For this review, take the finished solid that the model builds, in its own axes (mm). Face numbers are marked on the shaded views. A direction names the side the tool comes from. Round coordinates to 2 decimals unless told otherwise and drop trailing zeros. Order: outer loops, then holes, each group sorted by start corner. A loop starts at its lowest first (then second) coordinate and runs counter-clockwise, first axis right, second up. Notation, with made-up numbers: M 84.25,-30.5 L 132.25,-30.5 A19 cw 132.25,-24.5 Z; hole C 30.5,48.25 d10. An arc over 180 degrees is marked long. Put each result on its own line as item: value.
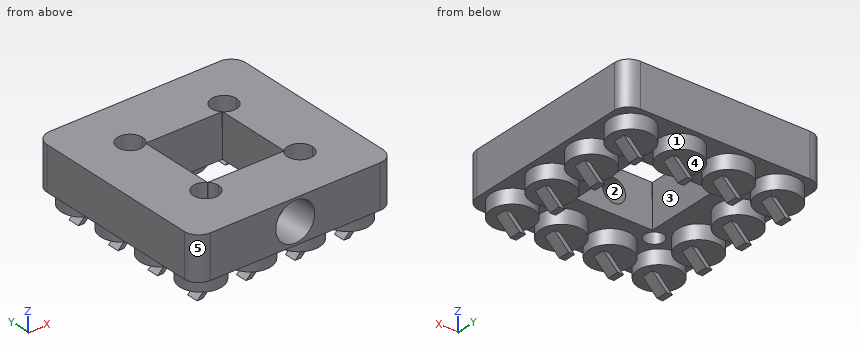
Autodesk Inventor part; units mm, degrees
ref_plane "YZ Plane" through (0, 0, 0) normal (1, 0, 0) x (0, 1, 0)
ref_plane "XZ Plane" through (0, 0, 0) normal (0, 1, 0) x (-1, 0, 0)
ref_plane "XY Plane" through (0, 0, 0) normal (0, 0, 1) x (1, 0, 0)
sketch "Sketch1" plane through (0, 0, 0) normal (0, 0, 1) x (1, 0, 0)
  circle A0 centre (16.335, -16.335) radius 2.25
  circle A1 centre (-16.335, 16.335) radius 2.25
  circle A2 centre (16.335, 16.335) radius 2.25
  circle A3 centre (-16.335, -16.335) radius 2.25
  line L0 (-13.335, 13.335) -> (13.335, 13.335)
  line L1 (13.335, 13.335) -> (13.335, -13.335)
  line L2 (13.335, -13.335) -> (-13.335, -13.335)
  line L3 (-13.335, -13.335) -> (-13.335, 13.335)
  circle A4 centre (25.5, -25.5) radius 8.0375
  circle A5 centre (8.5, -25.5) radius 8.0375
  circle A6 centre (-25.5, -25.5) radius 8.0375
  circle A7 centre (-8.5, -25.5) radius 8.0375
  circle A8 centre (25.5, -8.5) radius 8.0375
  circle A9 centre (25.5, 8.5) radius 8.0375
  circle A10 centre (-25.5, -8.5) radius 8.0375
  circle A11 centre (-25.5, 8.5) radius 8.0375
  circle A12 centre (25.5, 25.5) radius 8.0375
  circle A13 centre (8.5, 25.5) radius 8.0375
  circle A14 centre (-25.5, 25.5) radius 8.0375
  circle A15 centre (-8.5, 25.5) radius 8.0375
  arc A16 (29.5, -34.5) -> (34.5, -29.5) centre (29.5, -29.5) ccw
  line L4 (34.5, -29.5) -> (34.5, 29.5)
  arc A17 (34.5, 29.5) -> (29.5, 34.5) centre (29.5, 29.5) ccw
  line L5 (29.5, 34.5) -> (-29.5, 34.5)
  arc A18 (-29.5, 34.5) -> (-34.5, 29.5) centre (-29.5, 29.5) ccw
  line L6 (-34.5, 29.5) -> (-34.5, -29.5)
  arc A19 (-34.5, -29.5) -> (-29.5, -34.5) centre (-29.5, -29.5) ccw
  line L7 (-29.5, -34.5) -> (29.5, -34.5)
  circle A20 centre (-25.5, -25.5) radius 7.2875
  circle A21 centre (-8.5, -25.5) radius 7.2875
  circle A22 centre (8.5, -25.5) radius 7.2875
  circle A23 centre (25.5, -25.5) radius 7.2875
  circle A24 centre (-25.5, -8.5) radius 7.2875
  circle A25 centre (25.5, -8.5) radius 7.2875
  circle A26 centre (-25.5, 8.5) radius 7.2875
  circle A27 centre (25.5, 8.5) radius 7.2875
  circle A28 centre (-25.5, 25.5) radius 7.2875
  circle A29 centre (-8.5, 25.5) radius 7.2875
  circle A30 centre (8.5, 25.5) radius 7.2875
  circle A31 centre (25.5, 25.5) radius 7.2875
  point P0 (0, 0)
  dimension "d40" = 0.75
  dimension "d41" = 0.75
  dimension "d42" = 0.75
  dimension "d43" = 0.75
  dimension "d44" = 0.75
  dimension "d45" = 0.75
  dimension "d46" = 0.75
  dimension "d47" = 0.75
  dimension "d48" = 0.75
  dimension "d49" = 0.75
  dimension "d50" = 0.75
  dimension "d51" = 0.75
extrude "Extrusion1" add sketch "Sketch1" against normal blind 5 contours A20 | A21 | A22 | A23 | A24 | A25 | A26 | A27 | A28 | A29 | A30 | A31
ref_plane "Work Plane1" through (0, 0, 0) normal (0, 0, 1) x (1, 0, 0)
sketch "Sketch2" plane through (0, 0, 0) normal (0, 0, 1) x (1, 0, 0)
  circle A0 centre (16.335, -16.335) radius 2.25
  circle A1 centre (-16.335, 16.335) radius 2.25
  circle A2 centre (16.335, 16.335) radius 2.25
  circle A3 centre (-16.335, -16.335) radius 2.25
  line L0 (-13.335, 13.335) -> (13.335, 13.335)
  line L1 (13.335, 13.335) -> (13.335, -13.335)
  line L2 (13.335, -13.335) -> (-13.335, -13.335)
  line L3 (-13.335, -13.335) -> (-13.335, 13.335)
  circle A4 centre (25.5, -25.5) radius 8.0375
  circle A5 centre (8.5, -25.5) radius 8.0375
  circle A6 centre (-25.5, -25.5) radius 8.0375
  circle A7 centre (-8.5, -25.5) radius 8.0375
  circle A8 centre (25.5, -8.5) radius 8.0375
  circle A9 centre (25.5, 8.5) radius 8.0375
  circle A10 centre (-25.5, -8.5) radius 8.0375
  circle A11 centre (-25.5, 8.5) radius 8.0375
  circle A12 centre (25.5, 25.5) radius 8.0375
  circle A13 centre (8.5, 25.5) radius 8.0375
  circle A14 centre (-25.5, 25.5) radius 8.0375
  circle A15 centre (-8.5, 25.5) radius 8.0375
  arc A16 (29.5, -34.5) -> (34.5, -29.5) centre (29.5, -29.5) ccw
  line L4 (34.5, -29.5) -> (34.5, 29.5)
  arc A17 (34.5, 29.5) -> (29.5, 34.5) centre (29.5, 29.5) ccw
  line L5 (29.5, 34.5) -> (-29.5, 34.5)
  arc A18 (-29.5, 34.5) -> (-34.5, 29.5) centre (-29.5, 29.5) ccw
  line L6 (-34.5, 29.5) -> (-34.5, -29.5)
  arc A19 (-34.5, -29.5) -> (-29.5, -34.5) centre (-29.5, -29.5) ccw
  line L7 (-29.5, -34.5) -> (29.5, -34.5)
  circle A20 centre (-16.335, 16.335) radius 3.25
  circle A21 centre (16.335, 16.335) radius 3.25
  circle A22 centre (-16.335, -16.335) radius 3.25
  circle A23 centre (16.335, -16.335) radius 3.25
  point P0 (0, 0)
  dimension "d4" = 1
  dimension "d5" = 1
  dimension "d6" = 1
  dimension "d7" = 1
extrude "Extrusion2" add sketch "Sketch2" along normal blind 15 contours A4 | A5 | A6 | A7 | A8 | A9 | A10 | A11 | A12 | A13 | A14 | A15 | L7 A19 L6 A18 L5 A17 L4 A16
sketch "Sketch3" plane through (25.5, 25.5, -5) normal (0, 0, -1) x (-1, 0, 0)
  line L0 (-4.0375, 2.0375) -> (-2.0375, 2.0375)
  line L1 (-2.0375, 2.0375) -> (-2.0375, -2.0375)
  line L2 (-2.0375, -2.0375) -> (-4.0375, -2.0375)
  line L3 (-4.0375, -2.0375) -> (-4.0375, 2.0375)
  circle A0 centre (0, 0) radius 8.0375
  line L4 (12.165, -12.165) -> (38.835, -12.165)
  line L5 (12.165, -38.835) -> (12.165, -12.165)
  line L6 (12.9625, 2.0375) -> (14.9625, 2.0375)
  line L7 (14.9625, 2.0375) -> (14.9625, -2.0375)
  line L8 (14.9625, -2.0375) -> (12.9625, -2.0375)
  line L9 (12.9625, -2.0375) -> (12.9625, 2.0375)
  line L10 (29.9625, 2.0375) -> (31.9625, 2.0375)
  line L11 (31.9625, 2.0375) -> (31.9625, -2.0375)
  line L12 (31.9625, -2.0375) -> (29.9625, -2.0375)
  line L13 (29.9625, -2.0375) -> (29.9625, 2.0375)
  line L14 (46.9625, 2.0375) -> (48.9625, 2.0375)
  line L15 (48.9625, 2.0375) -> (48.9625, -2.0375)
  line L16 (48.9625, -2.0375) -> (46.9625, -2.0375)
  line L17 (46.9625, -2.0375) -> (46.9625, 2.0375)
  line L18 (-4.0375, -14.9625) -> (-2.0375, -14.9625)
  line L19 (-2.0375, -14.9625) -> (-2.0375, -19.0375)
  line L20 (-2.0375, -19.0375) -> (-4.0375, -19.0375)
  line L21 (-4.0375, -19.0375) -> (-4.0375, -14.9625)
  line L22 (12.9625, -14.9625) -> (14.9625, -14.9625)
  line L23 (14.9625, -14.9625) -> (14.9625, -19.0375)
  line L24 (14.9625, -19.0375) -> (12.9625, -19.0375)
  line L25 (12.9625, -19.0375) -> (12.9625, -14.9625)
  line L26 (29.9625, -14.9625) -> (31.9625, -14.9625)
  line L27 (31.9625, -14.9625) -> (31.9625, -19.0375)
  line L28 (31.9625, -19.0375) -> (29.9625, -19.0375)
  line L29 (29.9625, -19.0375) -> (29.9625, -14.9625)
  line L30 (46.9625, -14.9625) -> (48.9625, -14.9625)
  line L31 (48.9625, -14.9625) -> (48.9625, -19.0375)
  line L32 (48.9625, -19.0375) -> (46.9625, -19.0375)
  line L33 (46.9625, -19.0375) -> (46.9625, -14.9625)
  line L34 (-4.0375, -31.9625) -> (-2.0375, -31.9625)
  line L35 (-2.0375, -31.9625) -> (-2.0375, -36.0375)
  line L36 (-2.0375, -36.0375) -> (-4.0375, -36.0375)
  line L37 (-4.0375, -36.0375) -> (-4.0375, -31.9625)
  line L38 (12.9625, -31.9625) -> (14.9625, -31.9625)
  line L39 (14.9625, -31.9625) -> (14.9625, -36.0375)
  line L40 (14.9625, -36.0375) -> (12.9625, -36.0375)
  line L41 (12.9625, -36.0375) -> (12.9625, -31.9625)
  line L42 (29.9625, -31.9625) -> (31.9625, -31.9625)
  line L43 (31.9625, -31.9625) -> (31.9625, -36.0375)
  line L44 (31.9625, -36.0375) -> (29.9625, -36.0375)
  line L45 (29.9625, -36.0375) -> (29.9625, -31.9625)
  line L46 (46.9625, -31.9625) -> (48.9625, -31.9625)
  line L47 (48.9625, -31.9625) -> (48.9625, -36.0375)
  line L48 (48.9625, -36.0375) -> (46.9625, -36.0375)
  line L49 (46.9625, -36.0375) -> (46.9625, -31.9625)
  line L50 (-4.0375, -48.9625) -> (-2.0375, -48.9625)
  line L51 (-2.0375, -48.9625) -> (-2.0375, -53.0375)
  line L52 (-2.0375, -53.0375) -> (-4.0375, -53.0375)
  line L53 (-4.0375, -53.0375) -> (-4.0375, -48.9625)
  line L54 (12.9625, -48.9625) -> (14.9625, -48.9625)
  line L55 (14.9625, -48.9625) -> (14.9625, -53.0375)
  line L56 (14.9625, -53.0375) -> (12.9625, -53.0375)
  line L57 (12.9625, -53.0375) -> (12.9625, -48.9625)
  line L58 (29.9625, -48.9625) -> (31.9625, -48.9625)
  line L59 (31.9625, -48.9625) -> (31.9625, -53.0375)
  line L60 (31.9625, -53.0375) -> (29.9625, -53.0375)
  line L61 (29.9625, -53.0375) -> (29.9625, -48.9625)
  line L62 (46.9625, -48.9625) -> (48.9625, -48.9625)
  line L63 (48.9625, -48.9625) -> (48.9625, -53.0375)
  line L64 (48.9625, -53.0375) -> (46.9625, -53.0375)
  line L65 (46.9625, -53.0375) -> (46.9625, -48.9625)
  dimension "d9" = 2
  dimension "d10" = 6
  dimension "d11" = 6
  dimension "d12" = 4
  dimension "d15" = 17
  dimension "d18" = 17
sketch "Sketch4" plane through (8.5, 25.5, -5) normal (0, 0, -1) x (-1, 0, 0)
  point P0 (8.5, -25.5)
ref_plane "Work Plane2" through (-34.5, -34.5, -179.8) normal (0, -1, 0) x (1, 0, 0)
sketch "Sketch5" plane through (-34.5, -34.5, -179.8) normal (0, -1, 0) x (1, 0, 0)
  line L0 (62.0375, 174.8) -> (64.0375, 174.8)
  line L1 (62.0375, 174.8) -> (57.0375, 169.8)
  line L2 (62.0375, 174.8) -> (69.1086, 174.8) construction
  point P0 (34.5, 179.8)
  dimension "d21" = 135
  dimension "d23" = 5
sweep "Sweep1" add profiles "Sketch3" path "Sketch5" path curves L1 contours L0 L1 L2 L3 | L6 L7 L8 L9 | L10 L11 L12 L13 | L14 L15 L16 L17 | L18 L19 L20 L21 | L30 L31 L32 L33 | L34 L35 L36 L37 | L46 L47 L48 L49 | L50 L51 L52 L53 | L54 L55 L56 L57 | L58 L59 L60 L61 | L62 L63 L64 L65
sketch "Sketch6" plane through (-29.5, -34.5, 0) normal (0, -1, 0) x (1, 0, 0)
  circle A0 centre (29.5, 7.5) radius 6.75
  line L0 (59, 0) -> (0, 0)
  line L1 (64, 0) -> (64, 15)
  point P0 (29.5, 0)
  dimension "d26" = 7.5
  dimension "d27" = 13.5
  dimension "d28" = 34.5
extrude "Extrusion3" cut sketch "Sketch6" against normal blind 12
sketch "Sketch7" plane through (0, -22.5, 7.5) normal (0, -1, 0) x (1, 0, 0)
  circle A0 centre (0, 0) radius 6.75
  circle A1 centre (0, 0) radius 4
  point P0 (0, -7.5)
  dimension "d31" = 8
extrude "Extrusion4" cut sketch "Sketch7" against normal up to next contours A1
sketch "Sketch8" plane through (0, 0, 15) normal (0, 0, 1) x (1, 0, 0)
  circle A0 centre (16.335, 16.335) radius 3.25
  circle A1 centre (16.335, -16.335) radius 3.25
  circle A2 centre (-16.335, -16.335) radius 3.25
  circle A3 centre (-16.335, 16.335) radius 3.25
  circle A4 centre (16.335, 16.335) radius 4.35
  circle A5 centre (16.335, -16.335) radius 4.35
  circle A6 centre (-16.335, 16.335) radius 4.35
  circle A7 centre (-16.335, -16.335) radius 4.35
  point P0 (0, 0)
  dimension "d34" = 1.1
  dimension "d35" = 1.1
  dimension "d36" = 1.1
  dimension "d37" = 1.1
extrude "Extrusion5" cut sketch "Sketch8" against normal blind 5.2
properties part number "WeightCap"
(1) Add section A-A on z = 7.5. Give the boundary of the cut face in (x, y) (3 decimals).
A:
outline: M -34.5,-29.5 A5 ccw -29.5,-34.5 L -6.75,-34.5 L -6.75,-22.5 L -4,-22.5 L -4,-13.335 L -13.335,-13.335 L -13.335,13.335 L 13.335,13.335 L 13.335,-13.335 L 4,-13.335 L 4,-22.5 L 6.75,-22.5 L 6.75,-34.5 L 29.5,-34.5 A5 ccw 34.5,-29.5 L 34.5,29.5 A5 ccw 29.5,34.5 L -29.5,34.5 A5 ccw -34.5,29.5 Z; hole C -16.335,-16.335 d6.5; hole C -16.335,16.335 d6.5; hole C 16.335,-16.335 d6.5; hole C 16.335,16.335 d6.5
(2) Insertion check: pin 1 Ø4 at (x, z) = (-24, -8.5) entering from -Y; pin 2 Ø10 at (x, y) = (-2, 12.5) entering from -Z; pin 3 Ø2 at (x, y) = (-3, -20) entering from -Z; pin 4 Ø5 at (x, y) = (-16.335, 16.335) entering from +Z (3 decimals). Each pin has a flat end and moves straight along its axis. Give the tip position at first contact, or say it passes through.
A:
pin 1: stops at y = -27.54
pin 2: stops at z = 0
pin 3: stops at z = -5
pin 4: passes through
(3) For the marked faces 1, 2 and 3, list the 3-axis set-ups (+Z, -Z, +X, -X, +Y, -Y) from which the entire face can be reached by the end or side of a thin tool; tool diameter is ignored.
A:
face 1: -Z
face 2: -Y
face 3: +Z, -Z
(4) Add section D-D on x = -25.5. State how many separate pieces and enclosed holes the cut face has, then the cut area to 3 significant figures.
A:
separate pieces: 5
enclosed holes: 0
area: 1,360 mm2
(5) Draft analysis for pull direction Z (two halves, no side actions). For the marked faces 4 and 5, state which applies: released by +Z, released by -Z, zero draft, split by the parting line, or undercut.
A:
face 4: undercut
face 5: zero draft
(6) Add section C-C on y = 4. Give the boundary of the cut face in (x, z) (3 decimals), then the cut area to 3 significant figures.
A:
outline: M -34.5,0 L -31.232,0 L -31.232,-5 L -19.768,-5 L -19.768,0 L -13.335,0 L -13.335,15 L -34.5,15 Z; M 13.335,0 L 19.768,0 L 19.768,-5 L 31.232,-5 L 31.232,0 L 34.5,0 L 34.5,15 L 13.335,15 Z
area: 750 mm2
(7) To check wall thickness, follow L1, parallel to X at y = -26, z = -2.25; L2, parallel to Y at x = -16, z = 3.75; L3, parallel to X at y = -20, z = -3. State the ranges of each line that lie inside material, in increasing order.
A:
L1: x = -32.77 to -18.23, -15.77 to -1.23, 1.23 to 15.77, 18.23 to 32.77
L2: y = -34.5 to -19.57, -13.1 to 13.1, 19.57 to 34.5
L3: x = -30.28 to -20.72, -13.28 to -3.72, 3.72 to 13.28, 20.72 to 30.28
(8) Add section B-B on x = -8. Give the boundary of the cut face in (y, z) (1 decimal).
A:
outline: M -34.5,0 L -32.8,0 L -32.8,-5 L -18.2,-5 L -18.2,0 L -13.3,0 L -13.3,15 L -34.5,15 Z; M -27.5,-8.5 L -23.5,-8.5 L -23.5,-6.5 L -27.5,-6.5 Z; M 13.3,0 L 18.2,0 L 18.2,-5 L 32.8,-5 L 32.8,0 L 34.5,0 L 34.5,15 L 13.3,15 Z; M 23.5,-8.5 L 27.5,-8.5 L 27.5,-6.5 L 23.5,-6.5 Z
